Source: CAD feature listing. Evaluate the final solid. Frame: model axes, mm. Face numbers are marked on the shaded views. A direction names the side the tool comes from. Give positions to 0.01 mm unless a question says otherwise; leave off trailing zeros. Order: outer loops, then holes, each group sorted by start corner. A loop starts at its lowest first (then second) coordinate and runs counter-clockwise, first axis right, second up.
1) Section A-A, the plane x = -17.78. Return loops of the section in (y, z), plus the area to 3 significant figures.
2) Material intervals for line 1 (X direction, y = 1.6, z = 0); line 2 (X direction, y = 15, z = 13); line 3 (Y direction, x = -58, z = -1.5), sorted ascending.
3) Section B-B, the plane y = 26. Return loops of the section in (x, z).
4) Section D-D, the plane x = -61.5. Return loops of the section in (y, z).
5) First-contact query: P1, Ø2, axis at y = 28, z = -7.5, coming from the -X side; P2, Ø5, axis at y = 12, z = -0.5, coming from the -X side; P3, Ø6, axis at y = 24, z = 12, coming from the +X side. Flat tips, straight axial feed; report the tip coordinate or a pass-through.
6) Access query for the marked faces 1, 2 and 3. Directions: +Z, -Z, +X, -X, +Y, -Y. A direction counts if a zero-diameter tool reaches every point of the face in a straight line with its end or side. Return the directions, or none.
```python
from build123d import *

# Parameters (mm, degrees)
SKETCH3_W           = 114.3
SKETCH3_H           = 38.1
BOSS_EXTRUDE1_DEPTH = 3.81
SKETCH4_R           = 13.5453125
BOSS_EXTRUDE2_DEPTH = 19.05
FILLET1_R           = 2.032
SKETCH5_R           = 2.749999961
CUT_EXTRUDE4_DEPTH  = 12.7


with BuildPart() as part:
    # Sketch3 → Boss-Extrude1 (new body)
    with BuildSketch(Plane(origin=(0, 0, 0), x_dir=(1, 0, 0), z_dir=(0, 1, 0))):
        Rectangle(SKETCH3_W, SKETCH3_H)
    extrude(amount=BOSS_EXTRUDE1_DEPTH)

    # Sketch4 → Boss-Extrude2 (add, symmetric)
    with BuildSketch(Plane.XY):
        with BuildLine():
            Line((-36.071859255, 3.81), (36.071859255, 3.81))
            ThreePointArc((36.071859255, 3.81), (41.198342199, 6.412778013), (42.122274879, 12.087425946))
            ThreePointArc((42.122274879, 12.087425946), (41.806974837, 13.2052175), (41.567140999, 14.341594112))
            Line((41.567140999, 14.341594112), (45.319258538, 15.003193668))
            ThreePointArc((45.319258538, 15.003193668), (67.365546349, 6.979001129), (63.291557028, 30.083742702))
            ThreePointArc((63.291557028, 30.083742702), (61.010906137, 30.694841267), (58.658787305, 30.900625))
            Line((58.658787305, 30.900625), (58.658787305, 34.710625))
            ThreePointArc((58.658787305, 34.710625), (61.672505693, 34.446958806), (64.594653774, 33.663971588))
            ThreePointArc((64.594653774, 33.663971588), (75.750433611, 14.341594112), (58.658787305, 0))
            Line((58.658787305, 0), (-58.658787305, 0))
            ThreePointArc((-58.658787305, 0), (-70.930846463, 5.083253342), (-76.014099805, 17.3553125))
            ThreePointArc((-76.014099805, 17.3553125), (-55.993216901, 34.504703346), (-42.122274879, 12.087425946))
            ThreePointArc((-42.122274879, 12.087425946), (-41.198342199, 6.412778013), (-36.071859255, 3.81))
        make_face()
        with Locations(Location((-58.658787305, 17.3553125, 0), (0, 0, 180))):
            Circle(SKETCH4_R, mode=Mode.SUBTRACT)
    extrude(amount=BOSS_EXTRUDE2_DEPTH, both=True)

    # Fillet1
    # the kernel refuses this fillet: 2.032 mm, written as the material it takes off along each edge
    with BuildSketch(Plane(origin=(58.658787305, 34.710625, 0), x_dir=(0, -1, 0), z_dir=(0, 0, -1)), Plane(origin=(41.567140999, 14.341594112, 0), x_dir=(0.9848077530122078, 0.17364817766693208, 0), z_dir=(0, 0, 1))) as fillet1_piece_1:
        with BuildLine():
            CenterArc((2.16732771, -2.032), FILLET1_R, 90, 97.620348072)
            ThreePointArc((0.153273302, -2.301460275), (0.03836072, -1.153279249), (0, 0))
            Line((0, 0), (2.16732771, 0))
        make_face()
    extrude(amount=24.816396244, mode=Mode.SUBTRACT)
    with BuildSketch(Plane(origin=(58.658787305, 30.900625, 0), x_dir=(0.9978615634411592, -0.06536283505758803, 0), z_dir=(0, 0, -1)), Plane(origin=(45.319258538, 15.003193668, 0), x_dir=(0.23764666877900192, -0.9713516669148425, 0), z_dir=(0, 0, 1))) as fillet1_piece_2:
        with BuildLine():
            CenterArc((1.903537334, -2.027654697), FILLET1_R, 93.747686363, 82.504627273)
            Line((-0.124117363, -1.894837416), (0, 0))
            ThreePointArc((0, 0), (0.885360027, -0.028965791), (1.770720053, 0))
        make_face()
    extrude(amount=23.797245223, mode=Mode.SUBTRACT)
    with BuildSketch(Plane(origin=(45.319258538, 15.003193668, 0), x_dir=(-0.9848077530122076, -0.17364817766693288, 0), z_dir=(0, 0, -1)), Plane(origin=(58.658787305, 30.900625, 0), x_dir=(0, 1, 0), z_dir=(0, 0, 1))) as fillet1_piece_3:
        with BuildLine():
            CenterArc((1.898898089, -2.032), FILLET1_R, 90, 82.504627273)
            ThreePointArc((-0.115739283, -1.766933481), (-0.028965791, -0.885360027), (0, 0))
            Line((0, 0), (1.898898089, 0))
        make_face()
    extrude(amount=23.797245223, mode=Mode.SUBTRACT)
    with BuildSketch(Plane(origin=(41.567140999, 14.341594112, 0), x_dir=(0.23870589854739682, -0.9710919081110089, 0), z_dir=(0, 0, -1)), Plane(origin=(58.658787305, 34.710625, 0), x_dir=(0.9977896842762429, -0.06645107938864023, 0), z_dir=(0, 0, 1))) as fillet1_piece_4:
        with BuildLine():
            CenterArc((2.171529904, -2.027508638), FILLET1_R, 86.189825964, 97.620348072)
            Line((0.144021266, -2.162537232), (0, 0))
            ThreePointArc((0, 0), (1.153279249, 0.03836072), (2.306558498, 0))
        make_face()
    extrude(amount=24.816396244, mode=Mode.SUBTRACT)

    # Sketch5 → Cut-Extrude4 (cut)
    with BuildSketch(Plane(origin=(0, 3.81, 0), x_dir=(1, 0, 0), z_dir=(0, 1, 0))):
        with Locations(Location((-17.78, 0, 0), (0, 0, 270))):
            Circle(SKETCH5_R)
        with Locations(Location((3.81, 0, 0), (0, 0, 270))):
            Circle(SKETCH5_R)
    extrude(amount=-CUT_EXTRUDE4_DEPTH, mode=Mode.SUBTRACT)


solid = part.part
```
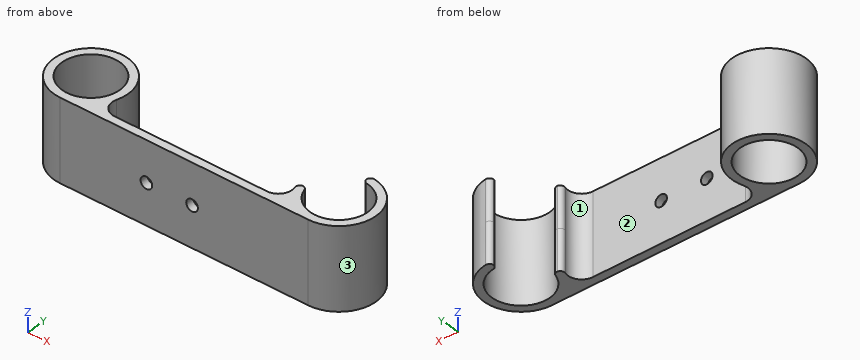
From the geometry:
1. outline: (0, -19.05) - (3.81, -19.05) - (3.81, -2.75) - (0, -2.75) - close; (0, 2.75) - (3.81, 2.75) - (3.81, 19.05) - (0, 19.05) - close
1. area: 124 mm2
2. line 1: x = -65.94 to -20.53, -15.03 to 1.06, 6.56 to 65.94
2. line 2: x = -75.85 to -72, -45.32 to -41.46, 72 to 75.85
2. line 3: y = 0 to 3.83, 30.88 to 34.7
3. outline: (-73.71, -19.05) - (-69.09, -19.05) - (-69.09, 19.05) - (-73.71, 19.05) - close; (-48.23, -19.05) - (-43.61, -19.05) - (-43.61, 19.05) - (-48.23, 19.05) - close; (69.09, -19.05) - (73.71, -19.05) - (73.71, 19.05) - (69.09, 19.05) - close
4. outline: (0.23, -19.05) - (4.11, -19.05) - (4.11, 19.05) - (0.23, 19.05) - close; (30.6, -19.05) - (34.48, -19.05) - (34.48, 19.05) - (30.6, 19.05) - close
5. P1: stops at x = -73.09
5. P2: stops at x = -75.78
5. P3: stops at x = 75.63
6. face 1: +Z, -Z
6. face 2: +Z, -Z, +Y
6. face 3: +Z, -Z, +X
